from build123d import *

# Parameters (mm, degrees)
SKETCH1_W           = 89
SKETCH1_H           = 24
BOSS_EXTRUDE1_DEPTH = 4
SKETCH2_R           = 1.6
CUT_EXTRUDE1_DEPTH  = 47.262836057
CHAMFER1_SIZE       = 0.7
SKETCH3_W           = 89
SKETCH3_H           = 6
CUT_EXTRUDE2_DEPTH  = 2.5
SKETCH4_W           = 89
SKETCH4_H           = 4
BOSS_EXTRUDE2_DEPTH = 3.39
SKETCH5_W           = 89
SKETCH5_H           = 4
BOSS_EXTRUDE3_DEPTH = 12.62


with BuildPart() as part:
    # Sketch1 → Boss-Extrude1 (new body)
    with BuildSketch(Plane(origin=(0, 0, 0), x_dir=(1, 0, 0), z_dir=(0, 1, 0))):
        Rectangle(SKETCH1_W, SKETCH1_H)
    extrude(amount=BOSS_EXTRUDE1_DEPTH)

    # Sketch2 → Cut-Extrude1 (cut, through all)
    with BuildSketch(Plane(origin=(0, 4, 0), x_dir=(1, 0, 0), z_dir=(0, 1, 0))):
        with Locations(Location((-40.6, 3.5, 0), (0, 0, 270))):
            Circle(SKETCH2_R)
        with Locations(Location((-40.6, -9.95, 0), (0, 0, 270))):
            Circle(SKETCH2_R)
        with Locations(Location((40.6, 3.5, 0), (0, 0, 270))):
            Circle(SKETCH2_R)
        with Locations(Location((40.6, -9.95, 0), (0, 0, 270))):
            Circle(SKETCH2_R)
    extrude(amount=-CUT_EXTRUDE1_DEPTH, mode=Mode.SUBTRACT)

    # Chamfer1
    # the kernel refuses this chamfer: 0.7 mm, written as the material it takes off along each edge
    with BuildSketch(Plane(origin=(40.6, 4, 9.95), x_dir=(0, 0, 1), z_dir=(-1, 0, 0))) as chamfer1_piece_1:
        Polygon((1.6 + CHAMFER1_SIZE, 0), (1.6, -CHAMFER1_SIZE), (1.6, 0), align=None)
    revolve(axis=Axis((40.6, 4, 9.95), (0, 1, 0)), mode=Mode.SUBTRACT)
    with BuildSketch(Plane(origin=(-40.6, 4, -3.5), x_dir=(0, 0, 1), z_dir=(-1, 0, 0))) as chamfer1_piece_2:
        Polygon((1.6 + CHAMFER1_SIZE, 0), (1.6, -CHAMFER1_SIZE), (1.6, 0), align=None)
    revolve(axis=Axis((-40.6, 4, -3.5), (0, 1, 0)), mode=Mode.SUBTRACT)
    with BuildSketch(Plane(origin=(40.6, 4, -3.5), x_dir=(0, 0, 1), z_dir=(-1, 0, 0))) as chamfer1_piece_3:
        Polygon((1.6 + CHAMFER1_SIZE, 0), (1.6, -CHAMFER1_SIZE), (1.6, 0), align=None)
    revolve(axis=Axis((40.6, 4, -3.5), (0, 1, 0)), mode=Mode.SUBTRACT)
    with BuildSketch(Plane(origin=(-40.6, 4, 9.95), x_dir=(0, 0, 1), z_dir=(-1, 0, 0))) as chamfer1_piece_4:
        Polygon((1.6 + CHAMFER1_SIZE, 0), (1.6, -CHAMFER1_SIZE), (1.6, 0), align=None)
    revolve(axis=Axis((-40.6, 4, 9.95), (0, 1, 0)), mode=Mode.SUBTRACT)

    # Sketch3 → Cut-Extrude2 (cut)
    with BuildSketch(Plane(origin=(0, 4, 0), x_dir=(1, 0, 0), z_dir=(0, 1, 0))):
        with Locations((0, -3.65)):
            Rectangle(SKETCH3_W, SKETCH3_H)
    extrude(amount=-CUT_EXTRUDE2_DEPTH, mode=Mode.SUBTRACT)

    # Sketch4 → Boss-Extrude2 (add)
    with BuildSketch(Plane(origin=(0, 0, -12), x_dir=(-1, 0, 0), z_dir=(0, 0, -1))):
        with Locations((0, 2)):
            Rectangle(SKETCH4_W, SKETCH4_H)
    extrude(amount=BOSS_EXTRUDE2_DEPTH)

    # Sketch5 → Boss-Extrude3 (add)
    with BuildSketch(Plane.XZ):
        with Locations((0, -13.39)):
            Rectangle(SKETCH5_W, SKETCH5_H)
    extrude(amount=BOSS_EXTRUDE3_DEPTH)


solid = part.part
Can you work these out from the model? Positions are in its coordinate system, mm. A direction names the side the tool comes from. Coordinates: 2 decimals unless noted, no trailing zeros. Write each loop counter-clockwise with the first axis right and the second up, starting at its lowest first coordinate (ties: lowest second). Pieces come first, ordered by that corner, then holes. Notation, with made-up numbers: M 58.5,27.5 L 91.5,27.5 A19 ccw 91.5,57.5 Z; hole C -28.75,70.5 d6. An arc over 180 degrees is marked long. Use one line per item in the form item = value.
Q1. I need wall thicknesses on line 1 along X through (y, z) = (1.15, -3.5); line 2 along Z through (x, y) = (-17.5, 2.75); line 3 along Y through (x, z) = (3.5, 3). Which ranges of each line are inside material? Lowest first, please. Write a range as from..to.
Model answer:
line_1 = -44.5..-42.2, -39..39, 42.2..44.5
line_2 = -15.39..0.65, 6.65..12
line_3 = 0..1.5
Q2. If we section it at C-C (x = -11): Write out the boundary of the cut face in (y, z), then the cut area to 3 significant figures.
Model answer:
outline = M -12.62,-15.39 L 4,-15.39 L 4,0.65 L 1.5,0.65 L 1.5,6.65 L 4,6.65 L 4,12 L 0,12 L 0,-11.39 L -12.62,-11.39 Z
area = 145 mm^2
Q3. If we section it at D-D (y = -6.5): Write out the boundary of the cut face in (x, z), then the cut area to 3 significant figures.
Model answer:
outline = M -44.5,-15.39 L 44.5,-15.39 L 44.5,-11.39 L -44.5,-11.39 Z
area = 356 mm^2
Q4. If we section it at A-A (z = 9.95): Write out the boundary of the cut face in (x, y), then the cut area to 3 significant figures.
Model answer:
outline = M -44.5,0 L -42.2,0 L -42.2,3.3 L -42.9,4 L -44.5,4 Z; M -39,0 L 39,0 L 39,3.3 L 38.3,4 L -38.3,4 L -39,3.3 Z; M 42.2,0 L 44.5,0 L 44.5,4 L 42.9,4 L 42.2,3.3 Z
area = 329 mm^2
Q5. If we section it at B-B (x = -40.6): Write out the boundary of the cut face in (y, z).
Model answer:
outline = M -12.62,-15.39 L 4,-15.39 L 4,-5.8 L 3.3,-5.1 L 0,-5.1 L 0,-11.39 L -12.62,-11.39 Z; M 0,-1.9 L 3.3,-1.9 L 4,-1.2 L 4,0.65 L 1.5,0.65 L 1.5,6.65 L 4,6.65 L 4,7.65 L 3.3,8.35 L 0,8.35 Z; M 0,11.55 L 3.3,11.55 L 3.75,12 L 0,12 Z
Q6. For P1, Ø6.5, axis at x = -11.5, y = -8.5, coming from the +Z side; P2, Ø5, axis at x = 40.6, z = -3.5, coming from the +Y side; P3, Ø1.8, axis at x = 16, z = 4.5, coming from the +Y side; P4, Ø7, axis at x = -5, z = 1, coming from the -Y side, each with a flat end and sliding along its axis, tell me the tip position at first contact or that it passes through.
Model answer:
P1 = -11.39
P2 = 4
P3 = 1.5
P4 = 0
Q7. For faces 1 (the flat face through (-1, 3, 6.65)), 2 (the cylindrical face through (-39.25, 1.67, -2.64)), 3 (the flat face through (1, 0, 0)), which set-ups out of +Z, -Z, +X, -X, +Y, -Y let a thin tool reach every point of the face, with its end or its side?
Model answer:
face_1 = +X, -X, +Y
face_2 = +Y, -Y
face_3 = +Z, +X, -X, -Y
Q8. We'd pull the mould along Z, two halves only. Please class faces 4 (the flat face through (-1, 4, 9)), 5 (the flat face through (-1, 3, 0.65)), 6 (the flat face through (-1, 2, 12)), 7 (the conical face through (-40.52, 3.41, 8.24)): +Z half, -Z half, draft (parallel to the pull), parting line (faces both ways), or undercut.
Model answer:
face_4 = draft
face_5 = undercut
face_6 = +Z half
face_7 = undercut
